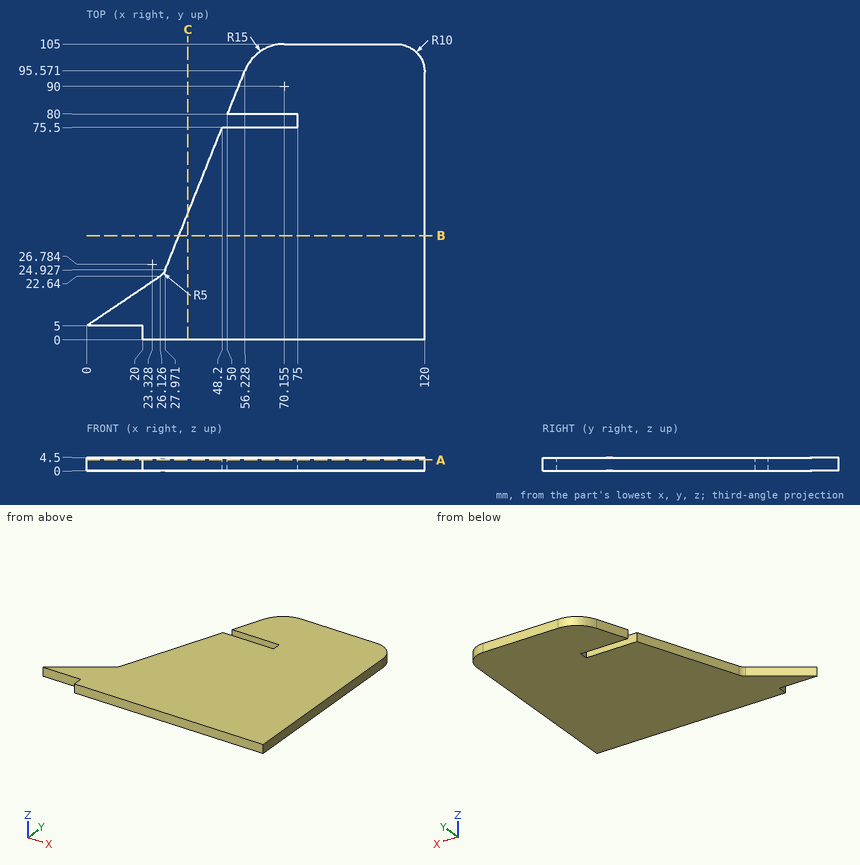
Geometry check sheet. Reference: drawing and pictorial views, mm from the part's lowest x, y, z. Give positions to 0.01 mm unless a question says otherwise; leave off trailing zeros. Order: outer loops, then holes, each group sorted by start corner. A loop starts at its lowest first (then second) coordinate and runs counter-clockwise, first axis right, second up. Notation, with made-up numbers: M 59,-16.5 L 117,-16.5 A33 ccw 117,13.5 Z; hole C 5.5,6 d8. An arc over 180 degrees is marked long. Answer in a Markdown table with one row per item.
1) Gauge pin test, flat ends, axial feed: P1, Ø1.3, axis at x = 65.5, z = 2.5, coming from the +Y side (1 decimal); P2, Ø1.5, axis at y = 93, z = 1, coming from the -X side; P3, Ø2, axis at y = 78, z = 2, coming from the -X side. Record the tip position at first contact, or that the pin passes through.
Filled sheet:
| item | result |
|---|---|
| P1 | stops at y = 104.5 |
| P2 | stops at x = 54.9 |
| P3 | stops at x = 75 |
2) Cross-section at B-B, the plane y = 37. Enter the section's corners in (x, z).
Filled sheet:
| item | result |
|---|---|
| outline | M 32.8,0 L 120,0 L 120,4.5 L 32.8,4.5 Z |
3) Cross-section at C-C, the plane x = 36. Enter the section's corners in (y, z).
Filled sheet:
| item | result |
|---|---|
| outline | M 0,0 L 45,0 L 45,4.5 L 0,4.5 Z |
4) Cross-section at A-A, the plane z = 3.75. Enter the section's corners in (x, y) (1 decimal), plus the area to 3 significant figures.
Filled sheet:
| item | result |
|---|---|
| outline | M 0,5 L 20,5 L 20,0 L 120,0 L 120,95 A10 ccw 110,105 L 70.2,105 A15 ccw 56.2,95.6 L 50,80 L 75,80 L 75,75.5 L 48.2,75.5 L 28,24.9 A5 cw 26.1,22.6 Z |
| area | 8,530 mm2 |
5) Thickness scan on L1, parallel to Y at x = 73.5, z = 0.55; L2, parallel to X at y = 79, z = 1.15; L3, parallel to Y at x = 68.5, z = 2.8. Record the ranges inside material, lowest first. Write a range as [from, to].
Filled sheet:
| item | result |
|---|---|
| L1 | y = [0, 75.5], [80, 105] |
| L2 | x = [75, 120] |
| L3 | y = [0, 75.5], [80, 104.91] |
